Drawing for the job (mm, zero at the part's lowest x, y, z). A direction names the side the tool comes from. Round coordinates to 2 decimals unless told otherwise and drop trailing zeros. Order: outer loops, then holes, each group sorted by start corner. A loop starts at its lowest first (then second) coordinate and runs counter-clockwise, first axis right, second up. Notation, with made-up numbers: M 33,66.25 L 84,66.25 A11 ccw 84,85.25 Z; hole C 25,50 d5. An arc over 180 degrees is marked long. Answer as CSV lines item,"result". Start each with the question number.
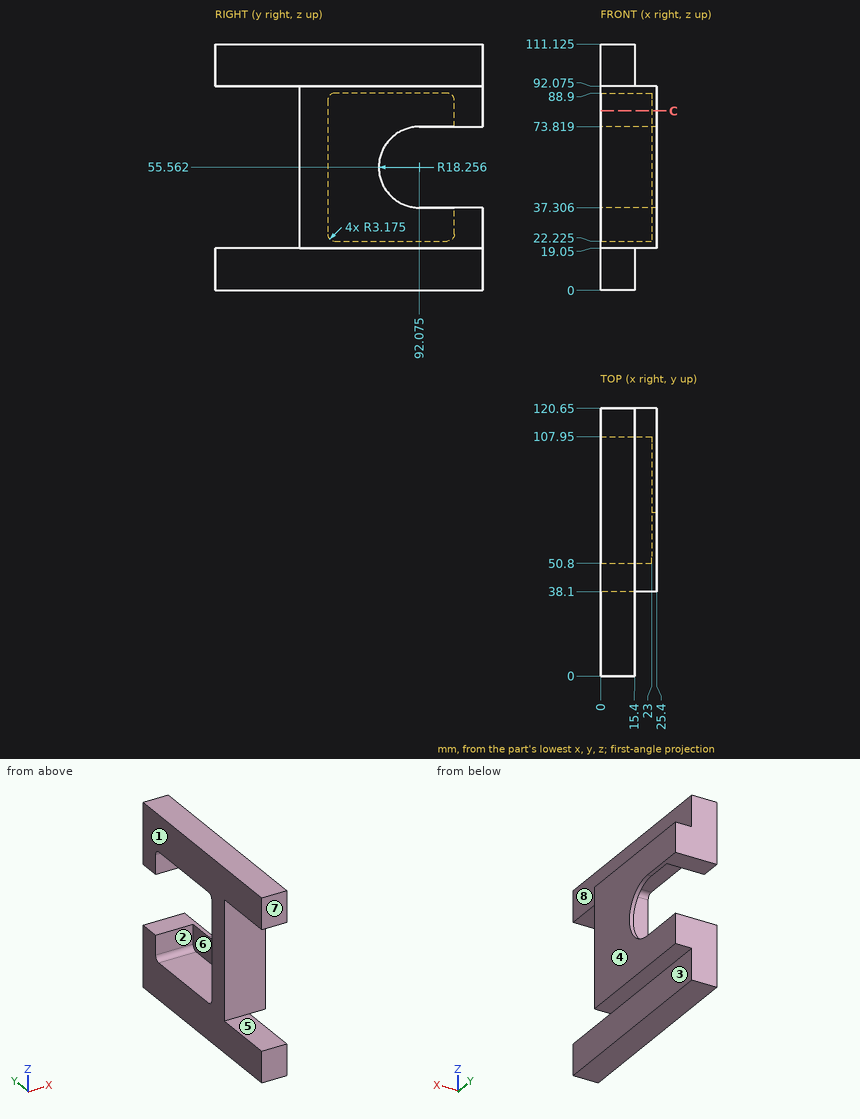
Q1. Band-saw the part on C-C, the plane z = 81. Write the cut outline in (x, y).
Q2. Drop flat-ended pins along their axis: P1, Ø9.5, axis at x = 11.5, z = 31, coming from the -Y side; P2, Ø3, axis at x = 20, y = 65.5, coming from the +Z side (1 decimal); P3, Ø3, axis at x = 4.5, y = 22.5, coming from the -Z side; P4, Ø7, axis at x = 7.5, z = 52.5, coming from the +Y side. Give the stop position or say it passes through.
Q3. Tool access for the marked faces 1, 2, 3, 4 and 5: list every direction of +Z, -Z, +X, -X, +Y, -Y with a clear straight run to the whole face (end or side of a thin tool).
Q4. Mould opens along Y. For the marked faces 6, 7 and 8 say: +Y half, -Y half, draft (parallel to the pull), parting line (faces both ways), or undercut.
Q5. Probe line 1 along Y through (x, z) = (5.25, 75.5); line 2 along Z through (x, y) = (3.5, 67) (1 decimal); line 3 along Y through (x, z) = (4, 38). List the from-to ranges inside material, lowest first. Write a range as from..to.
Answer:
1,outline,"M 0,38.1 L 25.4,38.1 L 25.4,120.65 L 0,120.65 L 0,107.95 L 23,107.95 L 23,50.8 L 0,50.8 Z"
2,P1,"stops at y = 38.1"
2,P2,"stops at z = 92.1"
2,P3,"stops at z = 0"
2,P4,"stops at y = 50.8"
3,face 1,"+Z, -Z, -X, +Y, -Y"
3,face 2,"-X"
3,face 3,"-Z, +X, +Y, -Y"
3,face 4,"+Z, -Z, +X, +Y, -Y"
3,face 5,"+X, -X, -Y"
4,face 6,"undercut"
4,face 7,"-Y half"
4,face 8,"draft"
5,line 1,"y = 38.1..50.8, 107.95..120.65"
5,line 2,"z = 0..22.2, 88.9..111.1"
5,line 3,"y = 38.1..50.8"
